The listing builds one solid part. Answer for the finished solid, in the listing's coordinates (mm). Face numbers are marked on the shaded views. A direction names the side the tool comes from. Coordinates: 2 decimals unless noted, no trailing zeros. Write each loop counter-clockwise with the first axis right and the second up, starting at its lowest first coordinate (ties: lowest second). Pieces come first, ordered by that corner, then holes.
from build123d import *

# Parameters (mm, degrees)
BOSS_EXTRUDE1_DEPTH       = 20
SKETCH2_W                 = 20
SKETCH2_H                 = 40
CUT_EXTRUDE1_DEPTH        = 142.509716981
SHELL1_T                  = -2
SHELL1_THICKNESS_2_FACE_W = 20
SHELL1_THICKNESS_2_FACE_H = 18
SHELL1_THICKNESS_2_DEPTH  = 3
SHELL1_THICKNESS_3_FACE_W = 18
SHELL1_THICKNESS_3_FACE_H = 20
SHELL1_THICKNESS_3_DEPTH  = 3
CUT_EXTRUDE14_REACH       = 110.167
SKETCH34_R                = 2.5
SKETCH3_W                 = 2.5
SKETCH3_H                 = 10
BOSS_EXTRUDE2_DEPTH       = 5
FILLET2_R                 = 5
CUT_EXTRUDE3_REACH        = 149.838
SKETCH6_R                 = 1.5
SKETCH21_R                = 2.5
SKETCH21_R_2              = 1.5
BOSS_EXTRUDE10_DEPTH      = 2.5
BOSS_EXTRUDE10_DRAFT      = 3
MIRROR7_COPY_1_SKETCH_R   = 2.5
MIRROR7_COPY_1_SKETCH_R_2 = 1.5
MIRROR7_COPY_1_DEPTH      = 2.5
MIRROR7_COPY_1_DRAFT      = 3
SKETCH26_W                = 5
SKETCH26_H                = 10
CUT_EXTRUDE8_DEPTH        = 2
SKETCH7_W                 = 2.5
SKETCH7_H                 = 10
BOSS_EXTRUDE4_DEPTH       = 5
FILLET4_R                 = 5
SKETCH22_R                = 2.5
BOSS_EXTRUDE11_DEPTH      = 2.5
BOSS_EXTRUDE11_TAPER      = 3
SKETCH23_R                = 1.5
CUT_EXTRUDE7_DEPTH        = 10
SKETCH27_W                = 5
SKETCH27_H                = 10
CUT_EXTRUDE9_DEPTH        = 2
SKETCH10_W                = 2.5
SKETCH10_H                = 10
BOSS_EXTRUDE6_DEPTH       = 5
FILLET6_R                 = 5
SKETCH28_R                = 2.5
BOSS_EXTRUDE12_DEPTH      = 2.5
BOSS_EXTRUDE12_TAPER      = 3
SKETCH29_R                = 1.5
CUT_EXTRUDE10_DEPTH       = 10
SKETCH30_W                = 5
SKETCH30_H                = 10
CUT_EXTRUDE11_DEPTH       = 2
SKETCH13_W                = 2.5
SKETCH13_H                = 10
BOSS_EXTRUDE8_DEPTH       = 5
FILLET8_R                 = 5
SKETCH31_R                = 2.5
BOSS_EXTRUDE13_DEPTH      = 2.5
BOSS_EXTRUDE13_TAPER      = 3
SKETCH32_R                = 1.5
CUT_EXTRUDE12_DEPTH       = 10
SKETCH33_W                = 5
SKETCH33_H                = 10
CUT_EXTRUDE13_DEPTH       = 2


with BuildPart() as part:
    # Sketch1 → Boss-Extrude1 (new body)
    with BuildSketch(Plane.XY):
        Polygon((58, 114), (58, 115), (80, 115), (80, 20), (60, 0), (0, 0), (-10, 25), (-10, 105), (11, 105), (11, 110), (12, 110), (34, 110), (34, 115), (35, 115), (57, 115), (57, 114), align=None)
    extrude(amount=BOSS_EXTRUDE1_DEPTH)

    # Sketch2 → Cut-Extrude1 (cut, through all)
    with BuildSketch(Plane.XY.offset(20)):
        with Locations((70, 45)):
            Rectangle(SKETCH2_W, SKETCH2_H)
    extrude(amount=-CUT_EXTRUDE1_DEPTH, mode=Mode.SUBTRACT)

    # Shell1
    shell1_openings = [part.faces().sort_by_distance(p)[0] for p in [
        (32.550473836, 58.500730419, 20),
    ]]
    offset(amount=SHELL1_T, openings=shell1_openings, kind=Kind.INTERSECTION)

    # Shell1 thickness 2 face (on inner face of the shell) → Shell1 thickness 2 (add)
    with BuildSketch(Plane(origin=(68, 23, 11), x_dir=(1, 0, 0), z_dir=(0, 1, 0))):
        Rectangle(SHELL1_THICKNESS_2_FACE_W, SHELL1_THICKNESS_2_FACE_H)
    extrude(amount=-SHELL1_THICKNESS_2_DEPTH)

    # Shell1 thickness 3 face (on inner face of the shell) → Shell1 thickness 3 (add)
    with BuildSketch(Plane(origin=(68, 67, 11), x_dir=(0, 0, -1), z_dir=(0, -1, 0))):
        Rectangle(SHELL1_THICKNESS_3_FACE_W, SHELL1_THICKNESS_3_FACE_H)
    extrude(amount=-SHELL1_THICKNESS_3_DEPTH)

    # Cut-Extrude14: up to this face of the body (flat: up to its plane)
    cut_extrude14_end = Plane(part.part.faces().sort_by_distance((67.585786438, 20, 11))[0])
    # Sketch34 → Cut-Extrude14 (cut, up to the picked face)
    with BuildSketch(Plane(origin=(0, 70, 0), x_dir=(1, 0, 0), z_dir=(0, 1, 0)), mode=Mode.PRIVATE) as cut_extrude14_sk1:
        with Locations(Location((70, -11, 0), (0, 0, 270))):
            Circle(SKETCH34_R)
    cut_extrude14_tool1 = split(extrude(cut_extrude14_sk1.sketch, amount=-CUT_EXTRUDE14_REACH, mode=Mode.PRIVATE), bisect_by=cut_extrude14_end, keep=Keep.BOTH, mode=Mode.PRIVATE)
    add(cut_extrude14_tool1.solids().sort_by(Axis((70, 70, 11), (0, -1, 0)))[0], mode=Mode.SUBTRACT)

    # Sketch3 → Boss-Extrude2 (add)
    with BuildSketch(Plane(origin=(0, 115, 0), x_dir=(1, 0, 0), z_dir=(0, 1, 0))):
        with Locations((65.25, -10)):
            Rectangle(SKETCH3_W, SKETCH3_H)
        with Locations((72.75, -10)):
            Rectangle(SKETCH3_W, SKETCH3_H)
    extrude(amount=BOSS_EXTRUDE2_DEPTH)

    # Fillet2
    fillet2_edges = [part.edges().sort_by_distance(p)[0] for p in [
        (65.25, 120, 5),
        (65.25, 120, 15),
        (72.75, 120, 5),
        (72.75, 120, 15),
    ]]
    fillet(fillet2_edges, radius=FILLET2_R - 0.0001)  # a hair under: the kernel refuses the full size

    # Cut-Extrude3: up to this face of the body (flat: up to its plane)
    cut_extrude3_end = Plane(part.part.faces().sort_by_distance((64, 117.122079053, 10))[0])
    # Sketch6 → Cut-Extrude3 (cut, up to the picked face)
    with BuildSketch(Plane(origin=(74, 0, 0), x_dir=(0, 0, -1), z_dir=(1, 0, 0)), mode=Mode.PRIVATE) as cut_extrude3_sk1:
        with Locations((-10, 117.5)):
            Circle(SKETCH6_R)
    cut_extrude3_tool1 = split(extrude(cut_extrude3_sk1.sketch, amount=-CUT_EXTRUDE3_REACH, mode=Mode.PRIVATE), bisect_by=cut_extrude3_end, keep=Keep.BOTH, mode=Mode.PRIVATE)
    add(cut_extrude3_tool1.solids().sort_by(Axis((74, 117.5, 10), (-1, 0, 0)))[0], mode=Mode.SUBTRACT)


with BuildPart() as boss_extrude10_tool:
    # Sketch21 → Boss-Extrude10 (with draft: the straight prism first)
    with BuildSketch(Plane(origin=(66.5, 0, 0), x_dir=(0, 0, -1), z_dir=(1, 0, 0))):
        with Locations((-10, 117.5)):
            Circle(SKETCH21_R)
        with Locations((-10, 117.5)):
            Circle(SKETCH21_R_2, mode=Mode.SUBTRACT)
    extrude(amount=BOSS_EXTRUDE10_DEPTH)
    # Boss-Extrude10: the draft: its side faces are tilted about the plane it starts from
    boss_extrude10_sides = [boss_extrude10_tool.faces().sort_by_distance(p)[0] for p in [
        (67.75, 117.5, 12.5),
        (67.75, 117.5, 11.5),
    ]]
    draft(boss_extrude10_sides, Plane(origin=(66.5, 0, 0), x_dir=(0, 0, -1), z_dir=(1, 0, 0)), BOSS_EXTRUDE10_DRAFT)


with BuildPart() as part_1:
    add(part.part)

    # Boss-Extrude10: add boss_extrude10_tool
    add(boss_extrude10_tool.part)


with BuildPart() as mirror7_copy_1_tool:
    # Mirror7 copy 1 sketch → Mirror7 copy 1 (with draft: the straight prism first)
    with BuildSketch(Plane(origin=(71.5, 0, 0), x_dir=(0, 0, -1), z_dir=(-1, 0, 0))):
        with Locations((-10, -117.5)):
            Circle(MIRROR7_COPY_1_SKETCH_R)
        with Locations((-10, -117.5)):
            Circle(MIRROR7_COPY_1_SKETCH_R_2, mode=Mode.SUBTRACT)
    extrude(amount=MIRROR7_COPY_1_DEPTH)
    # Mirror7 copy 1: the draft: its side faces are tilted about the plane it starts from
    mirror7_copy_1_sides = [mirror7_copy_1_tool.faces().sort_by_distance(p)[0] for p in [
        (70.25, 117.5, 12.5),
        (70.25, 117.5, 11.5),
    ]]
    draft(mirror7_copy_1_sides, Plane(origin=(71.5, 0, 0), x_dir=(0, 0, -1), z_dir=(-1, 0, 0)), MIRROR7_COPY_1_DRAFT)


with BuildPart() as part_2:
    add(part_1.part)

    # Mirror7 copy 1: add mirror7_copy_1_tool
    add(mirror7_copy_1_tool.part)

    # Sketch26 → Cut-Extrude8 (cut)
    with BuildSketch(Plane(origin=(0, 115, 0), x_dir=(1, 0, 0), z_dir=(0, 1, 0))):
        with Locations((69, -10)):
            Rectangle(SKETCH26_W, SKETCH26_H)
    extrude(amount=-CUT_EXTRUDE8_DEPTH, mode=Mode.SUBTRACT)

    # Sketch7 → Boss-Extrude4 (add)
    with BuildSketch(Plane(origin=(0, 115, 0), x_dir=(1, 0, 0), z_dir=(0, 1, 0))):
        with Locations((41.25, -10)):
            Rectangle(SKETCH7_W, SKETCH7_H)
        with Locations((48.75, -10)):
            Rectangle(SKETCH7_W, SKETCH7_H)
    extrude(amount=BOSS_EXTRUDE4_DEPTH)

    # Fillet4
    fillet4_edges = [part_2.edges().sort_by_distance(p)[0] for p in [
        (41.25, 120, 5),
        (41.25, 120, 15),
        (48.75, 120, 5),
        (48.75, 120, 15),
    ]]
    fillet(fillet4_edges, radius=FILLET4_R - 0.0001)  # a hair under: the kernel refuses the full size

    # Sketch22 → Boss-Extrude11 (add)
    with BuildSketch(Plane(origin=(42.5, 0, 0), x_dir=(0, 0, -1), z_dir=(1, 0, 0))):
        with Locations((-10, 117.5)):
            Circle(SKETCH22_R)
    boss_extrude11 = extrude(amount=BOSS_EXTRUDE11_DEPTH, taper=BOSS_EXTRUDE11_TAPER)

    # Mirror8: Boss-Extrude11 across plane
    add(boss_extrude11.mirror(Plane(origin=(45, 117.5, 10), x_dir=(0, 0, 1), z_dir=(1, 0, 0))))

    # Sketch23 → Cut-Extrude7 (cut)
    with BuildSketch(Plane(origin=(50, 0, 0), x_dir=(0, 0, -1), z_dir=(1, 0, 0))):
        with Locations((-10, 117.5)):
            Circle(SKETCH23_R)
    extrude(amount=-CUT_EXTRUDE7_DEPTH, mode=Mode.SUBTRACT)

    # Sketch27 → Cut-Extrude9 (cut)
    with BuildSketch(Plane(origin=(0, 115, 0), x_dir=(1, 0, 0), z_dir=(0, 1, 0))):
        with Locations((45, -10)):
            Rectangle(SKETCH27_W, SKETCH27_H)
    extrude(amount=-CUT_EXTRUDE9_DEPTH, mode=Mode.SUBTRACT)

    # Sketch10 → Boss-Extrude6 (add)
    with BuildSketch(Plane(origin=(0, 110, 0), x_dir=(1, 0, 0), z_dir=(0, 1, 0))):
        with Locations((19.25, -10)):
            Rectangle(SKETCH10_W, SKETCH10_H)
        with Locations((26.75, -10)):
            Rectangle(SKETCH10_W, SKETCH10_H)
    extrude(amount=BOSS_EXTRUDE6_DEPTH)

    # Fillet6
    fillet6_edges = [part_2.edges().sort_by_distance(p)[0] for p in [
        (19.25, 115, 15),
        (19.25, 115, 5),
        (26.75, 115, 5),
        (26.75, 115, 15),
    ]]
    fillet(fillet6_edges, radius=FILLET6_R - 0.0001)  # a hair under: the kernel refuses the full size

    # Sketch28 → Boss-Extrude12 (add)
    with BuildSketch(Plane(origin=(20.5, 0, 0), x_dir=(0, 0, -1), z_dir=(1, 0, 0))):
        with Locations((-10, 112.5)):
            Circle(SKETCH28_R)
    boss_extrude12 = extrude(amount=BOSS_EXTRUDE12_DEPTH, taper=BOSS_EXTRUDE12_TAPER)

    # Mirror9: Boss-Extrude12 across plane
    add(boss_extrude12.mirror(Plane(origin=(23, 112.5, 10), x_dir=(0, 0, 1), z_dir=(1, 0, 0))))

    # Sketch29 → Cut-Extrude10 (cut)
    with BuildSketch(Plane(origin=(28, 0, 0), x_dir=(0, 0, -1), z_dir=(1, 0, 0))):
        with Locations((-10, 112.5)):
            Circle(SKETCH29_R)
    extrude(amount=-CUT_EXTRUDE10_DEPTH, mode=Mode.SUBTRACT)

    # Sketch30 → Cut-Extrude11 (cut)
    with BuildSketch(Plane(origin=(0, 110, 0), x_dir=(1, 0, 0), z_dir=(0, 1, 0))):
        with Locations((23, -10)):
            Rectangle(SKETCH30_W, SKETCH30_H)
    extrude(amount=-CUT_EXTRUDE11_DEPTH, mode=Mode.SUBTRACT)

    # Sketch13 → Boss-Extrude8 (add)
    with BuildSketch(Plane(origin=(0, 105, 0), x_dir=(1, 0, 0), z_dir=(0, 1, 0))):
        with Locations((-2.75, -10)):
            Rectangle(SKETCH13_W, SKETCH13_H)
        with Locations((4.75, -10)):
            Rectangle(SKETCH13_W, SKETCH13_H)
    extrude(amount=BOSS_EXTRUDE8_DEPTH)

    # Fillet8
    fillet8_edges = [part_2.edges().sort_by_distance(p)[0] for p in [
        (-2.75, 110, 15),
        (-2.75, 110, 5),
        (4.75, 110, 5),
        (4.75, 110, 15),
    ]]
    fillet(fillet8_edges, radius=FILLET8_R - 0.0001)  # a hair under: the kernel refuses the full size

    # Sketch31 → Boss-Extrude13 (add)
    with BuildSketch(Plane(origin=(-1.5, 0, 0), x_dir=(0, 0, -1), z_dir=(1, 0, 0))):
        with Locations((-10, 107.5)):
            Circle(SKETCH31_R)
    boss_extrude13 = extrude(amount=BOSS_EXTRUDE13_DEPTH, taper=BOSS_EXTRUDE13_TAPER)

    # Mirror10: Boss-Extrude13 across plane
    add(boss_extrude13.mirror(Plane(origin=(1, 107.5, 10), x_dir=(0, 0, 1), z_dir=(1, 0, 0))))

    # Sketch32 → Cut-Extrude12 (cut)
    with BuildSketch(Plane(origin=(6, 0, 0), x_dir=(0, 0, -1), z_dir=(1, 0, 0))):
        with Locations((-10, 107.5)):
            Circle(SKETCH32_R)
    extrude(amount=-CUT_EXTRUDE12_DEPTH, mode=Mode.SUBTRACT)

    # Sketch33 → Cut-Extrude13 (cut)
    with BuildSketch(Plane(origin=(0, 105, 0), x_dir=(1, 0, 0), z_dir=(0, 1, 0))):
        with Locations((1, -10)):
            Rectangle(SKETCH33_W, SKETCH33_H)
    extrude(amount=-CUT_EXTRUDE13_DEPTH, mode=Mode.SUBTRACT)


solid = part_2.part
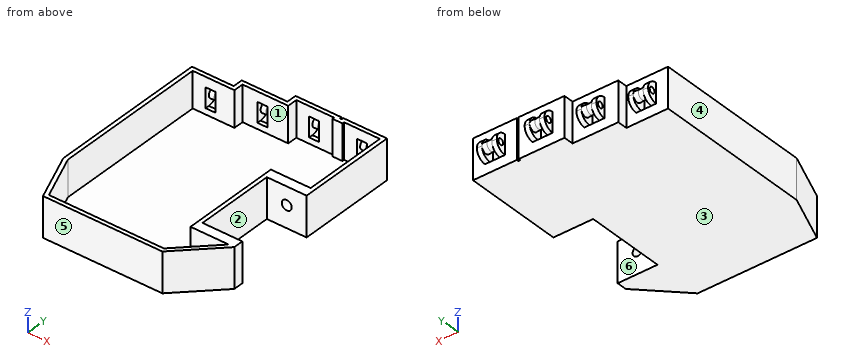
1. Flat-ended cylindrical pins translate along their axes: P1, Ø4, axis at y = 107.5, z = 9.5, coming from the -X side; P2, Ø4, axis at x = 52, z = 10.5, coming from the -Y side; P3, Ø3.5, axis at y = 117.5, z = 10, coming from the +X side; P4, Ø2, axis at x = 14, z = 13, coming from the +Y side. Find the tip coordinate at first contact, or state that the pin passes through.
Results found:
P1: stops at x = -4
P2: stops at y = 0
P3: stops at x = 74
P4: stops at y = 110
2. Section C-C on y = 117.5 is taken. State how many separate pieces and enclosed holes the cut face has, then the cut area to 3 significant figures.
Results found:
separate pieces: 4
enclosed holes: 0
area: 74.6 mm2
3. A tool of negligible diameter and unlimited length cuts with its end or side. For the marked faces 1, 2 and 3, from which of +Z, -Z, +X, -X, +Y, -Y can it reach the whole face along a straight path? Write none if from no direction.
Results found:
face 1: +Z
face 2: +Z, -Z, +X
face 3: -Z, +X, -X, +Y, -Y
4. Section A-A on x = 51.5 is taken. Give the vertices of the cut face in (y, z), then the cut area to 3 significant figures.
Results found:
outline: (0, 0) - (115, 0) - (115, 20) - (113, 20) - (113, 2) - (2, 2) - (2, 20) - (0, 20) - close
area: 302 mm2
5. For a pull along Y with two mould halves and no side action, classify the marked faces 4, 5 and 6 as pulls with the +Y half, pulls with the -Y half, needs draft (parallel to the pull), parting line crosses it, or undercut.
Results found:
face 4: needs draft
face 5: pulls with the -Y half
face 6: undercut
6. Section B-B on y = 49 is taken. Give the vertices of the cut face in (x, z).
Results found:
outline: (-10, 0) - (60, 0) - (60, 20) - (58, 20) - (58, 2) - (-8, 2) - (-8, 20) - (-10, 20) - close
7. Find the intervals of material crossed by L1, parallel to X at y = 66.2, z = 11; L2, parallel to X at y = 29, z = 14.5; L3, parallel to X at y = 79.5, z = 13, in increasing order.
Results found:
L1: x = -10 to -8, 58 to 67.5, 72.5 to 80
L2: x = -10 to -8, 58 to 60
L3: x = -10 to -8, 78 to 80
